Drawing for the job (mm, zero at the part's lowest x, y, z). A direction names the side the tool comes from. Give positions to 0.01 mm unless a question says otherwise; leave off trailing zeros. Loops run counter-clockwise (first coordinate to the right, second up) from the corner with the lowest first, then second, coordinate; pieces in that order, holes last. Notation, with made-up numbers: (45, 33) -> (50, 33) arc R27 ccw to (50, 69) -> close; hole circle Ø5 at (81.5, 25). An arc over 180 degrees is marked (long way). Answer in a Markdown table with one row per item. Add a question column.
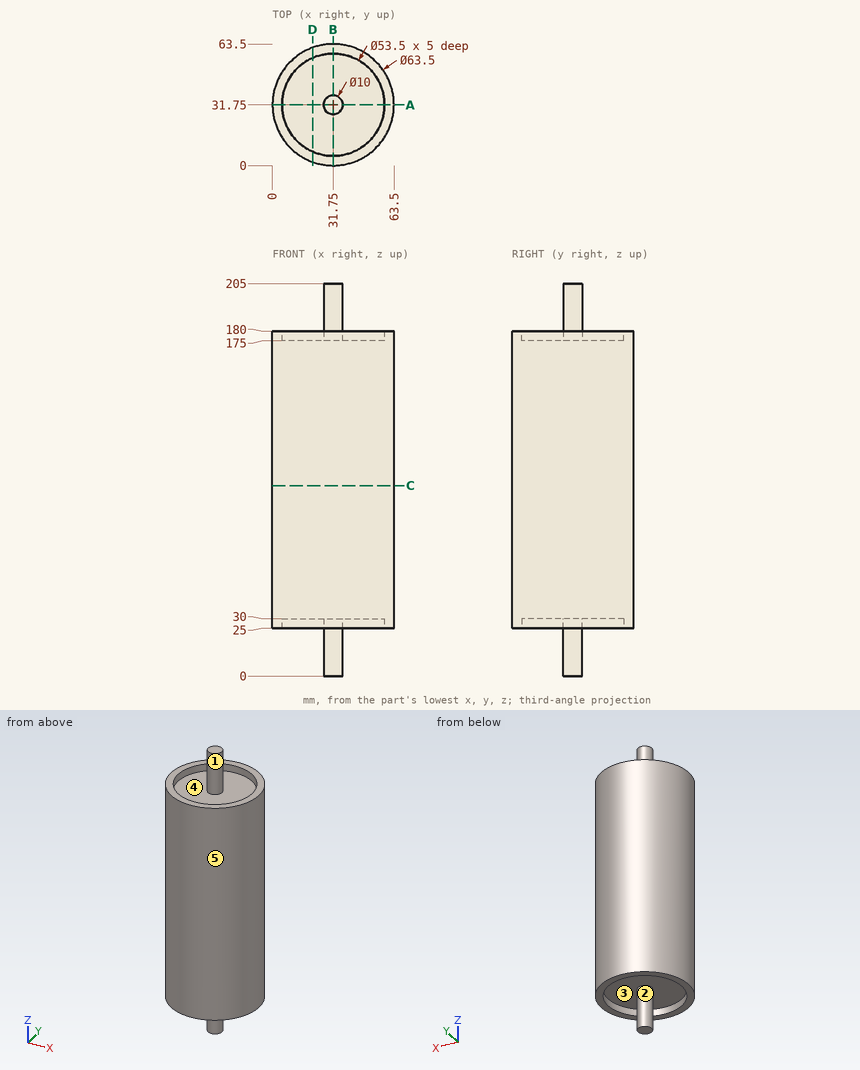
(1) Saw through at D-D, the plane x = 21. List the corners of the cut face in (y, z).
(2) Wall check: line 1 along Y through (x, z) = (31.75, 26.55); line 2 along X through (y, z) = (31, 176); line 3 along Z through (x, y) = (14, 10). Give the ranges that are in metal, low to high. Write a range as from..to.
(3) Saw through at C-C, the plane z = 99.5. List the corners of the cut face in (x, y).
(4) Saw through at A-A, the plane y = 31.75. List the corners of the cut face in (x, z).
(5) Two-plate mould, pull along X, no slides. Class the marked faces 3, 4 and 5: released by +X, released by -X, zero draft, split by the parting line, or undercut.
(6) Flat gauge pins, fed straight in: pin 1 Ø6 at (x, y) = (45.5, 44.5) entering from -Z; pin 2 Ø1 at (x, z) = (54.5, 143.5) entering from +Y; pin 3 Ø8 at (x, z) = (33.5, 41) entering from -Y. Where does each tip first touch, or does it go through?
(7) 3-axis set-ups, long thin cutter, end or side, ignore diameter. For the marked faces 1 and 2: which of +Z, -Z, +X, -X, +Y, -Y reach the whole face in a straight line?
Worked answers:
| question | item | result |
|---|---|---|
| 1 | outline | (1.88, 25) -> (7.26, 25) -> (7.26, 30) -> (56.24, 30) -> (56.24, 25) -> (61.62, 25) -> (61.62, 180) -> (56.24, 180) -> (56.24, 175) -> (7.26, 175) -> (7.26, 180) -> (1.88, 180) -> close |
| 2 | line 1 | 0..5, 26.75..36.75, 58.5..63.5 |
| 2 | line 2 | 0.01..5.01, 26.81..36.69, 58.49..63.49 |
| 2 | line 3 | 25..180 |
| 3 | outline | circle Ø63.5 at (31.75, 31.75) |
| 4 | outline | (0, 25) -> (5, 25) -> (5, 30) -> (26.75, 30) -> (26.75, 0) -> (36.75, 0) -> (36.75, 30) -> (58.5, 30) -> (58.5, 25) -> (63.5, 25) -> (63.5, 180) -> (58.5, 180) -> (58.5, 175) -> (36.75, 175) -> (36.75, 205) -> (26.75, 205) -> (26.75, 175) -> (5, 175) -> (5, 180) -> (0, 180) -> close |
| 5 | face 3 | undercut |
| 5 | face 4 | undercut |
| 5 | face 5 | split by the parting line |
| 6 | pin 1 | z = 30 |
| 6 | pin 2 | y = 54.4 |
| 6 | pin 3 | y = 0 |
| 7 | face 1 | +Z |
| 7 | face 2 | -Z |
